CAD build for the part. Positions are in the model's coordinates, mm. Coordinates: 2 decimals unless noted, no trailing zeros. Loops run counter-clockwise (first coordinate to the right, second up) from the corner with the lowest first, then second, coordinate; pieces in that order, holes last. Notation, with made-up numbers: (89.5, 80.5) -> (134.5, 80.5) arc R17 ccw to (134.5, 103.5) -> close; hole circle Ø1 at (59.5, 82). An arc over 180 degrees is marked (long way). Return JSON: item names as keys, results as strings. Group by question number.
(1) Saw through at C-C on x = -0.5. Write the cut outline in (y, z).
(2) Saw through at B-B on y = 0.3. Write the cut outline in (x, z), then the cut area to 3 significant figures.
(3) Saw through at A-A on z = 0. Write the cut outline in (x, y).
(4) Probe L1, parallel to Z at x = 0, y = 0.15; L2, parallel to Z at x = 5, y = 0.1; L3, parallel to X at y = 0.35, z = -5.25. List the from-to ranges inside material, lowest first.
(5) Mould opens along X. For faces 1 (the face through (4.5, 0.2, 3.5)), 2 (the face through (9.8, 0.2, -0.1)), 3 (the face through (-17, 0.5, 0)) say: pulls with the +X half, pulls with the -X half, needs draft (parallel to the pull), parting line crosses it, or undercut.
Autodesk Inventor part; units mm, degrees
ref_plane "YZ Plane" through (0, 0, 0) normal (1, 0, 0) x (0, 1, 0)
ref_plane "XZ Plane" through (0, 0, 0) normal (0, 1, 0) x (-1, 0, 0)
ref_plane "XY Plane" through (0, 0, 0) normal (0, 0, 1) x (1, 0, 0)
sketch "Sketch1" plane through (0, 0, 0) normal (0, 1, 0) x (-1, 0, 0)
  circle A0 centre (0, 0) radius 5.7
  arc A1 (0, 9) -> (0, -9) centre (0, 0) ccw construction
  line L0 (0, 9) -> (12.65, 9) construction
  line L1 (12.65, 9) -> (12.65, -9) construction
  line L2 (0, 0) -> (0, -9) construction
  line L3 (3.0786, -12.5) -> (30, -12.5)
  line L4 (35, -7.5) -> (35, 7.5)
  line L5 (30, 12.5) -> (3.0786, 12.5)
  arc A2 (35, 7.5) -> (30, 12.5) centre (30, 7.5) ccw
  arc A3 (30, -12.5) -> (35, -7.5) centre (30, -7.5) ccw
  arc A4 (-4.9268, 8.4715) -> (-4.9268, -8.4715) centre (0, 0) ccw
  line L6 (1.0676, -11.9578) -> (-4.9268, -8.4715)
  line L7 (1.0676, 11.9578) -> (-4.9268, 8.4715)
  arc A5 (1.0676, -11.9578) -> (3.0786, -12.5) centre (3.0786, -8.5) ccw
  arc A6 (3.0786, 12.5) -> (1.0676, 11.9578) centre (3.0786, 8.5) ccw
  point P0 (35, -12.5)
  point P1 (35, 12.5)
  point P2 (2, -12.5)
  point P3 (2, 12.5)
  dimension "d0" = 11.4
  dimension "d1" = 9
  dimension "d2" = 12.65
  dimension "d5" = 25
  dimension "d6" = 5
  dimension "d10" = 25
  dimension "d11" = 19.6
  dimension "d12" = 4
extrude "Extrusion1" add sketch "Sketch1" along normal blind 0.5
properties part number "Laser-Pivot-Ringpull"
Geometry results:
{
 "1": {"outline": "(0, -11.63) -> (0.5, -11.63) -> (0.5, -5.68) -> (0, -5.68) -> close; (0, 5.68) -> (0.5, 5.68) -> (0.5, 11.63) -> (0, 11.63) -> close"},
 "2": {"outline": "(-35, -7.5) arc R5 ccw to (-30, -12.5) -> (-3.08, -12.5) arc R4 ccw to (-1.07, -11.96) -> (4.93, -8.47) arc R9.8 ccw to (4.93, 8.47) -> (-1.07, 11.96) arc R4 ccw to (-3.08, 12.5) -> (-30, 12.5) arc R5 ccw to (-35, 7.5) -> close; hole circle Ø11.4 at (0, 0)", "area": "916 mm²"},
 "3": {"outline": "(-35, 0) -> (-5.7, 0) -> (-5.7, 0.5) -> (-35, 0.5) -> close; (5.7, 0) -> (9.8, 0) -> (9.8, 0.5) -> (5.7, 0.5) -> close"},
 "4": {"L1": "-11.34 to -5.7, 5.7 to 11.34", "L2": "-8.43 to -2.74, 2.74 to 8.43", "L3": "-35 to -2.22, 2.22 to 8.28"},
 "5": {"face 1": "undercut", "face 2": "pulls with the +X half", "face 3": "needs draft"}
}
